Autodesk Fusion 360 part; units mm, degrees
sketch "Sketch1" plane through (0, 0, 0) normal (0, 0, 1) x (1, 0, 0)
  line L0 (57.5, -29) -> (-57.5, -29)
  line L1 (-57.5, -29) -> (-57.5, 29)
  line L2 (-57.5, 29) -> (57.5, 29)
  line L3 (57.5, 29) -> (57.5, -29)
  line L4 (57.5, -29) -> (-57.5, 29) construction
  line L5 (-57.5, -29) -> (57.5, 29) construction
  line L6 (55.5, -27) -> (-55.5, -27)
  line L7 (-55.5, -27) -> (-55.5, 27)
  line L8 (-55.5, 27) -> (55.5, 27)
  line L9 (55.5, 27) -> (55.5, -27)
  line L10 (55.5, -27) -> (-55.5, 27) construction
  line L11 (-55.5, -27) -> (55.5, 27) construction
extrude "Extrude1" add sketch "Sketch1" along normal blind 2 contours L0 L1 L2 L3 | L6 L7 L8 L9
sketch "Sketch2" plane through (0, 0, 2) normal (0, 0, 1) x (-1, 0, 0)
  line L0 (-57.5, -29) -> (57.5, -29)
  line L1 (57.5, -29) -> (57.5, 29)
  line L2 (57.5, 29) -> (-57.5, 29)
  line L3 (-57.5, 29) -> (-57.5, -29)
  line L4 (-57.5, 29) -> (57.5, 29)
  line L5 (57.5, 29) -> (57.5, -29)
  line L6 (57.5, -29) -> (-57.5, -29)
  line L7 (-57.5, -29) -> (-57.5, 29)
  line L8 (-57.5, 29) -> (57.5, -29) construction
  line L9 (57.5, 29) -> (-57.5, -29) construction
  line L10 (-55.5, 27) -> (55.5, 27)
  line L11 (55.5, 27) -> (55.5, -27)
  line L12 (55.5, -27) -> (-55.5, -27)
  line L13 (-55.5, -27) -> (-55.5, 27)
  line L14 (-55.5, 27) -> (55.5, -27) construction
  line L15 (55.5, 27) -> (-55.5, -27) construction
extrude "Extrude2" add sketch "Sketch2" along normal blind 27
sketch "Sketch3" plane through (0, 0, 2) normal (0, 0, 1) x (-1, 0, 0)
  line L0 (55.5, -27) -> (55.5, 27)
  line L1 (55.5, 27) -> (-55.5, 27)
  line L2 (-55.5, 27) -> (-55.5, -27)
  line L3 (-55.5, -27) -> (55.5, -27)
  line L4 (-55.5, -27) -> (-29.5, -27)
  line L5 (-29.5, -27) -> (-29.5, 27)
  line L6 (-29.5, 27) -> (-55.5, 27)
  line L7 (-55.5, 27) -> (-55.5, -27)
  line L8 (-29.5, -27) -> (-27.5, -27)
  line L9 (-27.5, -27) -> (-27.5, 27)
  line L10 (-27.5, 27) -> (-29.5, 27)
  line L11 (-29.5, 27) -> (-29.5, -27)
extrude "Extrude3" add sketch "Sketch3" along normal blind 27 contours L1 L3 L5 L8 L9 L10 L11
sketch "Sketch4" plane through (0, 0, 29) normal (0, 0, 1) x (-1, 0, 0)
  line L0 (-27.5, 27) -> (55.5, 27)
  line L1 (55.5, 27) -> (55.5, -27)
  line L2 (55.5, -27) -> (-27.5, -27)
  line L3 (-27.5, -27) -> (-27.5, 27)
  line L4 (-29.5, 27) -> (-29.5, -27)
  line L5 (-29.5, -27) -> (-55.5, -27)
  line L6 (-55.5, -27) -> (-55.5, 27)
  line L7 (-55.5, 27) -> (-29.5, 27)
  line L8 (-57.5, -29) -> (57.5, -29)
  line L9 (57.5, -29) -> (57.5, 29)
  line L10 (57.5, 29) -> (-57.5, 29)
  line L11 (-57.5, 29) -> (-57.5, -29)
  line L12 (-25, -25) -> (-32.1654, -25)
  line L13 (-32.1654, -25) -> (-32.1654, -19.6955)
  line L14 (-32.1654, -19.6955) -> (-25, -19.6955)
  line L15 (-25, -19.6955) -> (-25, -25)
extrude "Extrude4" cut sketch "Sketch4" against normal blind 15 contours L3 L12 L14 L15 | L3 L4 L12 L14 | L4 L12 L13 L14
CAD build for the part. Positions are in the model's coordinates, mm. A direction names the side the tool comes from. Coordinates: 2 decimals unless noted, no trailing zeros. Order: outer loops, then holes, each group sorted by start corner. A loop starts at its lowest first (then second) coordinate and runs counter-clockwise, first axis right, second up. Notation, with made-up numbers: (44.5, 58.25) -> (76.5, 58.25) arc R21 cw to (76.5, 68.25) -> close; hole circle Ø1 at (-9.75, 6.25). An arc over 180 degrees is marked (long way). Use one line per item in the form item = value. Start each with the question number.
1) Tool access for faces 5 (the flat face through (17, 28, 29)), 6 (the flat face through (55.5, 0, 15)): list every direction of +Z, -Z, +X, -X, +Y, -Y with a clear straight run to the whole face (end or side of a thin tool).
2) Band-saw the part on D-D on y = 22.5. Give the cut face in (x, z), then the cut area to 3 significant figures.
3) Band-saw the part on C-C on z = 7.75. Give the cut face in (x, y), then the cut area to 3 significant figures.
4) Drop flat-ended pins along their axis: pin 1 (13 mm diameter, centred on x = 45, y = -6, fed in from +Z); pin 2 (0.6 mm diameter, centred on x = 29, y = 21.5, fed in from +Z). Give the stop position or say it passes through.
5) Pull direction X, two halves, no side cores. Call faces 1 (the flat face through (-57.5, 0, 14)), 2 (the flat face through (1, 29, 14)), 3 (the flat face through (57.5, 0, 14)), 4 (the flat face through (27.5, 0, 15)): +X half, -X half, draft (parallel to the pull), parting line (faces both ways), or undercut.
6) Band-saw the part on B-B on x = -47. Give the cut face in (y, z), then the cut area to 3 significant figures.
7) Drill centre lines: L1, parallel to X at y = -14.5, z = 4.5; L2, parallel to Y at x = -47, z = 20.5; L3, parallel to Z at x = -11, y = -25. Where is each one in solid material? Low to high. Write a range as [from, to].
8) Band-saw the part on A-A on z = 21.75. Give the cut face in (x, y).
Entries:
q1.face_5 = +Z, +X, -X, +Y, -Y
q1.face_6 = +Z
q2.outline = (-57.5, 0) -> (57.5, 0) -> (57.5, 29) -> (55.5, 29) -> (55.5, 2) -> (29.5, 2) -> (29.5, 14) -> (27.5, 14) -> (27.5, 2) -> (-55.5, 2) -> (-55.5, 29) -> (-57.5, 29) -> close
q2.area = 362 mm2
q3.outline = (-57.5, -29) -> (57.5, -29) -> (57.5, 29) -> (-57.5, 29) -> close; hole (-55.5, -27) -> (27.5, -27) -> (27.5, 27) -> (-55.5, 27) -> close; hole (29.5, -27) -> (55.5, -27) -> (55.5, 27) -> (29.5, 27) -> close
q3.area = 784 mm2
q4.pin_1 = 2
q4.pin_2 = 14
q5.face_1 = -X half
q5.face_2 = draft
q5.face_3 = +X half
q5.face_4 = undercut
q6.outline = (-29, 0) -> (29, 0) -> (29, 29) -> (27, 29) -> (27, 2) -> (-27, 2) -> (-27, 29) -> (-29, 29) -> close
q6.area = 224 mm2
q7.L1 = [-57.5, -55.5], [27.5, 29.5], [55.5, 57.5]
q7.L2 = [-29, -27], [27, 29]
q7.L3 = [0, 2]
q8.outline = (-57.5, -29) -> (57.5, -29) -> (57.5, 29) -> (-57.5, 29) -> close; hole (-55.5, -27) -> (27.5, -27) -> (27.5, 19.7) -> (29.5, 19.7) -> (29.5, -27) -> (55.5, -27) -> (55.5, 27) -> (29.5, 27) -> (29.5, 25) -> (27.5, 25) -> (27.5, 27) -> (-55.5, 27) -> close
